from build123d import *

# Parameters (mm, degrees)
BOSS_EXTRUDE1_DEPTH            = 10
SKETCH2_R                      = 5
CUT_EXTRUDE1_DEPTH             = 11
FILLET1_R                      = 3
CUT_EXTRUDE4_DEPTH             = 11
CUT_EXTRUDE5_DEPTH             = 8
FILLET2_R                      = 3
SKETCH7_R                      = 1.5
CUT_EXTRUDE6_DEPTH             = 10
M3X0_5_TAPPED_HOLE1_AT_2_COUNT = 2
M3X0_5_TAPPED_HOLE1_AT_2_PITCH = 40
M3X0_5_TAPPED_HOLE2_AT_2_COUNT = 2
M3X0_5_TAPPED_HOLE2_AT_2_PITCH = 40


with BuildPart() as part:
    # Sketch1 → Boss-Extrude1 (new body)
    with BuildSketch(Plane(origin=(0, 0, 0), x_dir=(1, 0, 0), z_dir=(0, 1, 0))):
        Polygon((0, 88), (0, 8), (8, 0), (88, 0), (96, 8), (96, 88), (88, 96), (8, 96), align=None)
    extrude(amount=BOSS_EXTRUDE1_DEPTH)

    # Sketch2 → Cut-Extrude1 (cut, through all)
    with BuildSketch(Plane(origin=(0, 0, 0), x_dir=(-1, 0, 0), z_dir=(0, -1, 0))):
        with BuildLine():
            Line((-45.411809549, 57.659258263), (-19.071067812, 84))
            Line((-19.071067812, 84), (-76.928932188, 84))
            Line((-76.928932188, 84), (-50.588190451, 57.659258263))
            ThreePointArc((-50.588190451, 57.659258263), (-48, 58), (-45.411809549, 57.659258263))
        make_face()
        with BuildLine():
            Line((-12, 76.928932188), (-38.340741737, 50.588190451))
            ThreePointArc((-38.340741737, 50.588190451), (-38.085551386, 49.305261922), (-38, 48))
            ThreePointArc((-38, 48), (-38.085551386, 46.694738078), (-38.340741737, 45.411809549))
            Line((-38.340741737, 45.411809549), (-12, 19.071067812))
            Line((-12, 19.071067812), (-12, 76.928932188))
        make_face()
        with BuildLine():
            Line((-19.071067812, 12), (-45.411809549, 38.340741737))
            ThreePointArc((-45.411809549, 38.340741737), (-48, 38), (-50.588190451, 38.340741737))
            Line((-50.588190451, 38.340741737), (-76.928932188, 12))
            Line((-76.928932188, 12), (-19.071067812, 12))
        make_face()
        with BuildLine():
            ThreePointArc((-57.659258263, 45.411809549), (-58, 48), (-57.659258263, 50.588190451))
            Line((-57.659258263, 50.588190451), (-84, 76.928932188))
            Line((-84, 76.928932188), (-84, 19.071067812))
            Line((-84, 19.071067812), (-57.659258263, 45.411809549))
        make_face()
        with Locations((-48, 48)):
            Circle(SKETCH2_R)
    extrude(amount=-CUT_EXTRUDE1_DEPTH, mode=Mode.SUBTRACT)

    # Fillet1
    fillet1_edges = [part.edges().sort_by_distance(p)[0] for p in [
        (50.588190451, 5, -38.340741737),
        (45.411809549, 5, -38.340741737),
        (19.071067812, 5, -12),
        (76.928932188, 5, -12),
        (38.340741737, 5, -45.411809549),
        (38.340741737, 5, -50.588190451),
        (12, 5, -76.928932188),
        (12, 5, -19.071067812),
        (57.659258263, 5, -50.588190451),
        (57.659258263, 5, -45.411809549),
        (84, 5, -19.071067812),
        (84, 5, -76.928932188),
        (45.411809549, 5, -57.659258263),
        (50.588190451, 5, -57.659258263),
        (76.928932188, 5, -84),
        (19.071067812, 5, -84),
    ]]
    fillet(fillet1_edges, radius=FILLET1_R)

    # Sketch5 → Cut-Extrude4 (cut, through all)
    with BuildSketch(Plane(origin=(0, 10, 0), x_dir=(1, 0, 0), z_dir=(0, 1, 0))):
        Polygon((8, 0), (8, 20.5), (0, 20.5), (0, 8), align=None)
        Polygon((96, 8), (88, 0), (88, 20.5), (96, 20.5), align=None)
        Polygon((96, 75.5), (88, 75.5), (88, 96), (96, 88), align=None)
        Polygon((8, 96), (8, 75.5), (0, 75.5), (0, 88), align=None)
    extrude(amount=-CUT_EXTRUDE4_DEPTH, mode=Mode.SUBTRACT)

    # Sketch6 → Cut-Extrude5 (cut)
    with BuildSketch(Plane(origin=(0, 10, 0), x_dir=(1, 0, 0), z_dir=(0, 1, 0))):
        Polygon((86, 73.5), (86, 94), (10, 94), (10, 73.5), (2, 73.5), (2, 22.5), (10, 22.5), (10, 2), (86, 2), (86, 22.5), (94, 22.5), (94, 73.5), align=None)
    extrude(amount=-CUT_EXTRUDE5_DEPTH, mode=Mode.SUBTRACT)

    # Fillet2
    fillet2_edges = [part.edges().sort_by_distance(p)[0] for p in [
        (8, 5, -75.5),
        (88, 5, -75.5),
        (88, 5, -20.5),
        (8, 5, -20.5),
        (94, 6, -73.5),
        (94, 6, -22.5),
        (86, 6, -2),
        (10, 6, -2),
        (2, 6, -22.5),
        (2, 6, -73.5),
        (10, 6, -94),
        (86, 6, -94),
    ]]
    fillet(fillet2_edges, radius=FILLET2_R)

    # Sketch7 → Cut-Extrude6 (cut)
    with BuildSketch(Plane.XZ):
        with Locations((78, -18)):
            Circle(SKETCH7_R)
        with Locations((18, -18)):
            Circle(SKETCH7_R)
        with Locations((18, -78)):
            Circle(SKETCH7_R)
        with Locations((78, -78)):
            Circle(SKETCH7_R)
    extrude(amount=-CUT_EXTRUDE6_DEPTH, mode=Mode.SUBTRACT)

    # Sketch13 → M3x0.5 Tapped Hole1 (revolve, cut)
    with BuildSketch(Plane(origin=(28, 6, 0), x_dir=(0, -1, 0), z_dir=(1, 0, 0))):
        Polygon((0, 0), (0, 8.251075774), (1.25, 7.5), (1.25, 0), align=None)
    m3x0_5_tapped_hole1 = revolve(axis=Axis((28, 6, 6.35), (0, 0, -1)), mode=Mode.SUBTRACT)

    # M3x0.5 Tapped Hole1 at 2: M3x0.5 Tapped Hole1 ×2
    with Locations(*[(i * M3X0_5_TAPPED_HOLE1_AT_2_PITCH, 0, 0) for i in range(1, M3X0_5_TAPPED_HOLE1_AT_2_COUNT)]):
        add(m3x0_5_tapped_hole1, mode=Mode.SUBTRACT)

    # Sketch15 → M3x0.5 Tapped Hole2 (revolve, cut)
    with BuildSketch(Plane(origin=(0, 6, -68), x_dir=(0, 0, 1), z_dir=(0, 1, 0))):
        Polygon((0, 0), (0, 8.251075774), (1.25, 7.5), (1.25, 0), align=None)
    m3x0_5_tapped_hole2 = revolve(axis=Axis((-6.35, 6, -68), (1, 0, 0)), mode=Mode.SUBTRACT)

    # M3x0.5 Tapped Hole2 at 2: M3x0.5 Tapped Hole2 ×2
    with Locations(*[(0, 0, i * M3X0_5_TAPPED_HOLE2_AT_2_PITCH) for i in range(1, M3X0_5_TAPPED_HOLE2_AT_2_COUNT)]):
        add(m3x0_5_tapped_hole2, mode=Mode.SUBTRACT)

    # Mirror1: M3x0.5 Tapped Hole1 across plane
    add(m3x0_5_tapped_hole1.mirror(Plane.XY.offset(-48)), mode=Mode.SUBTRACT)

    # Mirror1 copy 1 sketch → Mirror1 copy 1 (revolve, cut)
    with BuildSketch(Plane(origin=(68, 6, -96), x_dir=(0, -1, 0), z_dir=(1, 0, 0))):
        Polygon((0, 0), (0, -8.251075774), (1.25, -7.5), (1.25, 0), align=None)
    revolve(axis=Axis((68, 6, -102.35), (0, 0, -1)), mode=Mode.SUBTRACT)

    # Mirror2: M3x0.5 Tapped Hole2 across plane
    add(m3x0_5_tapped_hole2.mirror(Plane.ZY.offset(-48)), mode=Mode.SUBTRACT)

    # Mirror2 copy 1 sketch → Mirror2 copy 1 (revolve, cut)
    with BuildSketch(Plane(origin=(96, 6, -28), x_dir=(0, 0, 1), z_dir=(0, 1, 0))):
        Polygon((0, 0), (0, -8.251075774), (1.25, -7.5), (1.25, 0), align=None)
    revolve(axis=Axis((102.35, 6, -28), (1, 0, 0)), mode=Mode.SUBTRACT)


solid = part.part
Input: part model. Units: mm. Frame: model coordinates. A direction names the side the tool comes from. Round coordinates to 2 decimals unless told otherwise and drop trailing zeros. Order: outer loops, then holes, each group sorted by start corner. A loop starts at its lowest first (then second) coordinate and runs counter-clockwise, first axis right, second up. Notation, with made-up numbers: (77, -7) - (107, -7) arc R13 ccw to (107, -2) - close; hole circle Ø11 at (8.5, -24). An arc over 180 degrees is marked (long way). Answer as a JSON object with one key per item and string values. Group by question number.
(1) Draft query along X for faces 1 (the face through (47, 5, 0)), 2 (the face through (79.43, 0.99, -17.55)), 3 (the face through (0, 5, -48)). Return one class per face: released by +X, released by -X, zero draft, split by the parting line, or undercut.
(2) Reachability of faces 4 (the face through (68.97, 0.99, -34.1)), 5 (the face through (48, 6, -2)), 6 (the face through (27.95, 7.25, -95.01)), 7 (the face through (3, 5, -20.5)) from +Z, -Z, +X, -X, +Y, -Y: full face, straight path, thin tool, end or side. Return the list, or none.
(3) Cut plane A-A (x = 28). Return loops of the section in (y, z), then the cut area to 3 significant figures.
(4) Cut plane D-D (y = 6). Count the separate pieces of the cut face and the enclosed holes in it, then the cut area to 3 significant figures.
(5) Cut plane C-C (z = -68). Return loops of the section in (x, y).
(6) Material intervals for probe 1 along X at (y, z) = (9.75, -6.5); probe 2 along Y at (x, z) = (0.75, -28); probe 3 along X at (y, z) = (7, -42.5), sorted ascending. Write a range as from..to.
(7) Pin query (flat end, axial travel): P1, Ø1, axis at y = 6.5, z = -12, coming from the +X side; P2, Ø10, axis at x = 63.5, z = -83, coming from the +Y side. Return the tip coordinate at first contact, or that it passes through.
(8) Cut plane B-B (z = -87). Return loops of the section in (x, y), then the cut area to 3 significant figures.
Here are the results:
{
 "1": {"face 1": "zero draft", "face 2": "undercut", "face 3": "released by -X"},
 "2": {"face 4": "+Y, -Y", "face 5": "+Y", "face 6": "+Z, -Z", "face 7": "+Z, -X, +Y, -Y"},
 "3": {"outline": "(0, -96) - (4.75, -96) - (4.75, -94) - (2, -94) - (2, -84) - (0, -84) - close; (0, -75.07) - (2, -75.07) - (2, -60.93) - (0, -60.93) - close; (0, -35.07) - (2, -35.07) - (2, -20.93) - (0, -20.93) - close; (0, -12) - (2, -12) - (2, -2) - (4.75, -2) - (4.75, 0) - (0, 0) - close; (7.25, -96) - (10, -96) - (10, -94) - (7.25, -94) - close; (7.25, -2) - (10, -2) - (10, 0) - (7.25, 0) - close", "area": "127 mm^2"},
 "4": {"separate pieces": "8", "enclosed holes": "0", "area": "735 mm^2"},
 "5": {"outline": "(0, 0) - (12, 0) - (12, 2) - (2, 2) - (2, 4.75) - (0, 4.75) - close; (0, 7.25) - (2, 7.25) - (2, 10) - (0, 10) - close; (20.93, 0) - (35.07, 0) - (35.07, 2) - (20.93, 2) - close; (60.93, 0) - (75.07, 0) - (75.07, 2) - (60.93, 2) - close; (84, 0) - (96, 0) - (96, 4.75) - (94, 4.75) - (94, 2) - (84, 2) - close; (94, 7.25) - (96, 7.25) - (96, 10) - (94, 10) - close"},
 "6": {"probe 1": "x = 8..10, 86..88", "probe 2": "y = 0..4.75, 7.25..10", "probe 3": "x = 0..2, 94..96"},
 "7": {"P1": "stops at x = 88", "P2": "stops at y = 2"},
 "8": {"outline": "(8, 0) - (88, 0) - (88, 10) - (86, 10) - (86, 2) - (10, 2) - (10, 10) - (8, 10) - close", "area": "192 mm^2"}
}
